Verification items for the finished model (mm, model axes). Face numbers are marked on the shaded views. A direction names the side the tool comes from. Give positions to 0.01 mm unless a question says otherwise; leave off trailing zeros. Loops run counter-clockwise (first coordinate to the right, second up) from the corner with the lowest first, then second, coordinate; pieces in that order, holes last. Notation, with made-up numbers: (4, -35) - (17, -35) arc R9 ccw to (17, -31) - close; hole circle Ø10 at (83.25, 87.5). An arc over 180 degrees is marked (long way). Answer in a Markdown table with one row per item.
```python
from build123d import *

# Parameters (mm, degrees)
BOSS_EXTRU_1_DEPTH      = 2
BOSS_EXTRU_2_START      = -7
BOSS_EXTRU_2_DEPTH      = 5
BOSS_EXTRU_3_START      = -1
BOSS_EXTRU_3_DEPTH      = 1
CONG_1_R                = 0.25
BOSS_EXTRU_4_DEPTH      = 2
CONG_4_R                = 1
ESQUISSE5_R             = 5
ENL_V_MAT_EXTRU_1_DEPTH = 55.929567647
ESQUISSE6_W             = 15
ESQUISSE6_H             = 5
ENL_V_MAT_EXTRU_2_DEPTH = 2
ENL_V_MAT_EXTRU_3_DEPTH = 2


with BuildPart() as part:
    # Esquisse1 → Boss.-Extru.1 (new body)
    with BuildSketch(Plane.XY):
        with BuildLine():
            Line((31.551874669, -39.37254902), (31.551874669, 5.62745098))
            ThreePointArc((31.551874669, 5.62745098), (-28.41563861, 22.999431705), (12.980446097, -23.736555864))
            ThreePointArc((12.980446097, -23.736555864), (15.388180878, -23.882439984), (16.551874669, -25.995325621))
            Line((16.551874669, -25.995325621), (16.551874669, -39.37254902))
            Line((16.551874669, -39.37254902), (31.551874669, -39.37254902))
        make_face()
    extrude(amount=BOSS_EXTRU_1_DEPTH)



with BuildPart() as body_2:
    # Esquisse2 → Boss.-Extru.2 (new body)
    with BuildSketch(Plane.XY.offset(2).offset(BOSS_EXTRU_2_START)):
        with BuildLine():
            Line((14.551874669, -41.37254902), (33.551874669, -41.37254902))
            Line((33.551874669, -41.37254902), (33.551874669, 5.62745098))
            ThreePointArc((33.551874669, 5.62745098), (-30.105947119, 24.068476672), (13.837588955, -25.54357167))
            ThreePointArc((13.837588955, -25.54357167), (14.319135911, -25.572748494), (14.551874669, -25.995325621))
            Line((14.551874669, -25.995325621), (14.551874669, -41.37254902))
        make_face()
        with BuildLine():
            Line((16.551874669, -39.37254902), (31.551874669, -39.37254902))
            Line((31.551874669, -39.37254902), (31.551874669, 5.62745098))
            ThreePointArc((31.551874669, 5.62745098), (-28.41563861, 22.999431705), (12.980446097, -23.736555864))
            ThreePointArc((12.980446097, -23.736555864), (15.388180878, -23.882439984), (16.551874669, -25.995325621))
            Line((16.551874669, -25.995325621), (16.551874669, -39.37254902))
        make_face(mode=Mode.SUBTRACT)
    extrude(amount=BOSS_EXTRU_2_DEPTH)

    # Esquisse3 → Boss.-Extru.3 (add)
    with BuildSketch(Plane(origin=(0, 0, -5), x_dir=(-1, 0, 0), z_dir=(0, 0, -1)).offset(BOSS_EXTRU_3_START)):
        with BuildLine():
            ThreePointArc((-12.980446097, -23.736555864), (28.41563861, 22.999431705), (-31.551874669, 5.62745098))
            Line((-31.551874669, 5.62745098), (-31.051874669, 5.62745098))
            ThreePointArc((-31.051874669, 5.62745098), (27.993061483, 22.732170463), (-12.766160383, -23.284801913))
            Line((-12.766160383, -23.284801913), (-12.980446097, -23.736555864))
        make_face()
    extrude(amount=-BOSS_EXTRU_3_DEPTH)

    # Congé1
    cong_1_edges = [body_2.edges().sort_by_distance(p)[0] for p in [
        (-27.993061483, 22.732170463, -4),
    ]]
    fillet(cong_1_edges, radius=CONG_1_R)


with BuildPart() as part_1:
    add(part.part)

    add(body_2.part)  # Boss.-Extru.4 merges body 2
    # Esquisse4 → Boss.-Extru.4 (add)
    with BuildSketch(Plane.XY):
        with BuildLine():
            Line((14.551874669, -25.995325621), (14.551874669, -41.37254902))
            Line((14.551874669, -41.37254902), (33.551874669, -41.37254902))
            Line((33.551874669, -41.37254902), (33.551874669, 5.62745098))
            ThreePointArc((33.551874669, 5.62745098), (-30.105947119, 24.068476672), (13.837588955, -25.54357167))
            ThreePointArc((13.837588955, -25.54357167), (14.319135911, -25.572748494), (14.551874669, -25.995325621))
        make_face()
    extrude(amount=BOSS_EXTRU_4_DEPTH)

    # Congé4
    cong_4_edges = [part_1.edges().sort_by_distance(p)[0] for p in [
        (14.319135911, -25.572748494, 2),
        (14.551874669, -33.68393732, 2),
        (33.551874669, -17.87254902, 2),
        (-30.105947119, 24.068476672, 2),
    ]]
    fillet(cong_4_edges, radius=CONG_4_R)

    # Esquisse5 → Enlèv. mat.-Extru.1 (cut, through all)
    with BuildSketch(Plane.XY.offset(2)):
        with Locations((-0.948125331, 5.62745098)):
            Circle(ESQUISSE5_R)
    extrude(amount=-ENL_V_MAT_EXTRU_1_DEPTH, mode=Mode.SUBTRACT)

    # Esquisse6 → Enlèv. mat.-Extru.2 (cut)
    with BuildSketch(Plane.XZ.offset(41.37254902)):
        with Locations((24.051874669, -2.5)):
            Rectangle(ESQUISSE6_W, ESQUISSE6_H)
    extrude(amount=-ENL_V_MAT_EXTRU_2_DEPTH, mode=Mode.SUBTRACT)

    # Esquisse7 → Enlèv. mat.-Extru.3 (cut)
    with BuildSketch(Plane.XZ.offset(41.37254902)):
        with BuildLine():
            Line((14.551874669, -5), (16.551874669, -5))
            Line((16.551874669, -5), (16.551874669, 0))
            Line((16.551874669, 0), (31.551874669, 0))
            Line((31.551874669, 0), (31.551874669, -5))
            Line((31.551874669, -5), (33.551874669, -5))
            Line((33.551874669, -5), (33.551874669, 1))
            ThreePointArc((33.551874669, 1), (33.25898145, 1.707106781), (32.551874669, 2))
            Line((32.551874669, 2), (15.551874669, 2))
            ThreePointArc((15.551874669, 2), (14.844767888, 1.707106781), (14.551874669, 1))
            Line((14.551874669, 1), (14.551874669, -5))
        make_face()
    extrude(amount=-ENL_V_MAT_EXTRU_3_DEPTH, mode=Mode.SUBTRACT)


solid = part_1.part
```
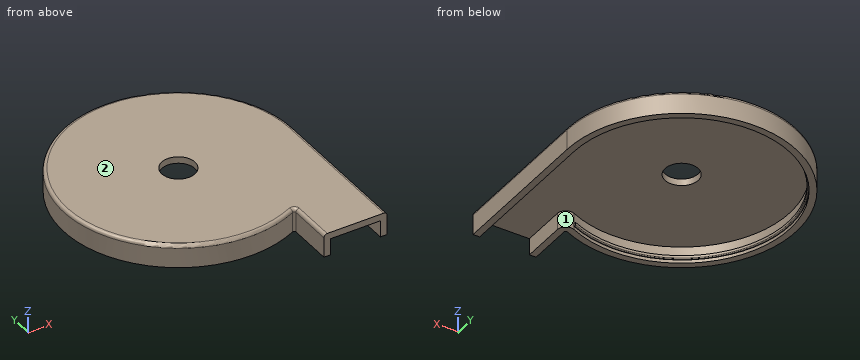
Q1. Go/stop test with flat-tipped pins: P1, Ø16, axis at x = -0.95, y = 5.63, coming from the +Z side; P2, Ø1.8, axis at y = -32.5, z = -3, coming from the -X side; P3, Ø3, axis at x = -3.5, z = -3, coming from the -Y side; P4, Ø1, axis at y = 25, z = -4, coming from the +X side. Record where each tip stops, or that it passes through.
Completed:
| item | result |
|---|---|
| P1 | z = 2 |
| P2 | x = 14.55 |
| P3 | y = -28.86 |
| P4 | x = 27.93 |
Q2. Tool access check on the marked faces 1 and 2. Record the directions out of +Z, -Z, +X, -X, +Y, -Y that give a thin tool (end or side, any length) a straight path to the whole face; none if there is none.
Completed:
| item | result |
|---|---|
| face 1 | -Z |
| face 2 | +Z, +X, -X, +Y, -Y |
Q3. Sectioned sample at B-B (z = -1.5). Record the cut outline in (x, y), and give its area (3 significant figures).
Completed:
| item | result |
|---|---|
| outline | (12.98, -23.74) arc R32.5 cw (long way) to (31.55, 5.63) - (31.55, -39.37) - (33.55, -39.37) - (33.55, 5.63) arc R34.5 ccw (long way) to (13.84, -25.54) arc R0.5 cw to (14.55, -26) - (14.55, -39.37) - (16.55, -39.37) - (16.55, -26) arc R2.5 ccw to start |
| area | 468 mm^2 |
Q4. Thickness scan on line 1 (X direction, y = -32, z = -3.5); line 2 (Z direction, x = 17, y = -10.5); line 3 (X direction, y = 27.5, z = -2.75). Record the ranges inside material, lowest first.
Completed:
| item | result |
|---|---|
| line 1 | 14.55 to 16.55, 31.55 to 33.55 |
| line 2 | 0 to 2 |
| line 3 | -27.63 to -24.99, 23.09 to 25.73 |
Q5. Sectioned sample at A-A (y = -33.5). Record the cut outline in (x, z).
Completed:
| item | result |
|---|---|
| outline | (14.55, -5) - (16.55, -5) - (16.55, 0) - (31.55, 0) - (31.55, -5) - (33.55, -5) - (33.55, 1) arc R1 ccw to (32.55, 2) - (15.55, 2) arc R1 ccw to (14.55, 1) - close |
